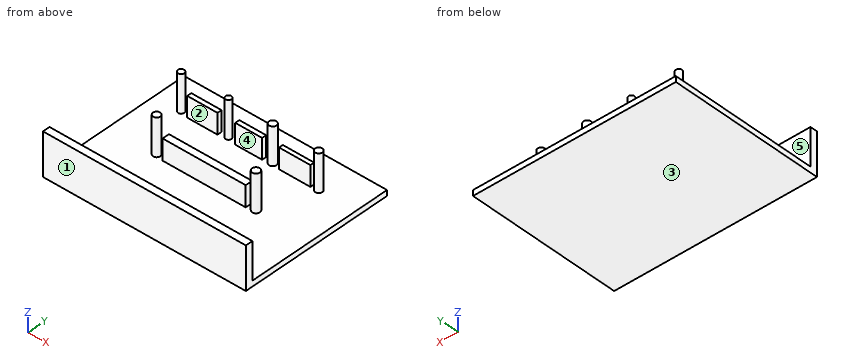
```python
from build123d import *

# Parameters (mm, degrees)
F0_W      = 138.621978
F0_H      = 105.59459
F1_DEPTH  = 3.81
F2_R      = 2.106167
F3_DEPTH  = 25.4
F4_R      = 2.000792
F5_DEPTH  = 25.4
F6_R      = 2.558459
F7_DEPTH  = 25.4
F8_R      = 2.472435
F9_DEPTH  = 25.4
F10_W     = 138.621978
F10_H     = 4.884328
F11_DEPTH = 25.4
F12_R     = 2.472435
F13_DEPTH = 25.4
F14_R     = 2.6519
F15_DEPTH = 25.4
F16_W     = 20.700261
F16_H     = 3.023634
F16_W_2   = 18.374391
F16_W_3   = 21.398022
F16_H_2   = 2.791049
F17_DEPTH = 13.97
F18_W     = 56.751281
F18_H     = 4.768038
F19_DEPTH = 14.224


with BuildPart() as f1:
    # F0 (on Top) → F1 (new body)
    with BuildSketch(Plane.XY):
        with Locations((1.744408, 1.046643)):
            Rectangle(F0_W, F0_H)
    extrude(amount=F1_DEPTH)

    # F2 (on face) → F3 (join)
    with BuildSketch(Plane.XY.offset(3.81)):
        with Locations((-49.192194, 31.515568)):
            Circle(F2_R)
    extrude(amount=F3_DEPTH)

    # F4 (on face) → F5 (join)
    with BuildSketch(Plane.XY.offset(3.81)):
        with Locations((-17.09516, 31.748157)):
            Circle(F4_R)
    extrude(amount=F5_DEPTH)

    # F6 (on face) → F7 (join)
    with BuildSketch(Plane.XY.offset(3.81)):
        with Locations((13.606353, 31.28298)):
            Circle(F6_R)
    extrude(amount=F7_DEPTH)

    # F8 (on face) → F9 (join)
    with BuildSketch(Plane.XY.offset(3.81)):
        with Locations((45.703389, 30.585218)):
            Circle(F8_R)
    extrude(amount=F9_DEPTH)

    # F10 (on face) → F11 (join)
    with BuildSketch(Plane.XY.offset(3.81)):
        with Locations((1.744408, -49.308488)):
            Rectangle(F10_W, F10_H)
    extrude(amount=F11_DEPTH)

    # F12 (on face) → F13 (join)
    with BuildSketch(Plane.XY.offset(3.81)):
        with Locations((-34.5392, -2.90734)):
            Circle(F12_R)
    extrude(amount=F13_DEPTH)

    # F14 (on face) → F15 (join)
    with BuildSketch(Plane.XY.offset(3.81)):
        with Locations((33.376262, -2.90734)):
            Circle(F14_R)
    extrude(amount=F15_DEPTH)

    # F16 (on face) → F17 (join)
    with BuildSketch(Plane.XY.offset(3.81)):
        with Locations((-33.027384, 31.166687)):
            Rectangle(F16_W, F16_H)
        with Locations((-1.395523, 31.166687)):
            Rectangle(F16_W_2, F16_H)
        with Locations((30.120045, 31.050394)):
            Rectangle(F16_W_3, F16_H_2)
    extrude(amount=F17_DEPTH)

    # F18 (on face) → F19 (join)
    with BuildSketch(Plane.XY.offset(3.81)):
        with Locations((-0.34888, -2.384019)):
            Rectangle(F18_W, F18_H)
    extrude(amount=F19_DEPTH)


solid = f1.part
```
Build history of the part. All positions in model axes, mm. Face numbers are marked on the shaded views. A direction names the side the tool comes from. Round coordinates to 2 decimals unless told otherwise and drop trailing zeros. Write each loop counter-clockwise with the first axis right and the second up, starting at its lowest first coordinate (ties: lowest second). Pieces come first, ordered by that corner, then holes. Notation, with made-up numbers: (78, 88) -> (109, 88) arc R15 ccw to (109, 107) -> close; hole circle Ø1 at (-33.75, 32.25). An arc over 180 degrees is marked (long way). Put each result on its own line as item: value.
Item 1: Wall check: probe 1 along Y at (x, z) = (-25.5, 10); probe 2 along Y at (x, z) = (-11, 11.5); probe 3 along X at (y, z) = (-1, 13.75). Give the ranges that are in metal, low to high. Write a range as from..to.
Here are the results:
probe 1: y = -51.75..-46.87, -4.77..0, 29.65..32.68
probe 2: y = -51.75..-46.87, -4.77..0
probe 3: x = -36.11..-32.97, -28.72..28.03, 31.53..35.22
Item 2: Slice it at B-B, the plane x = -40.5. Give the cut face in (y, z).
Here are the results:
outline: (-51.75, 0) -> (53.84, 0) -> (53.84, 3.81) -> (32.68, 3.81) -> (32.68, 17.78) -> (29.65, 17.78) -> (29.65, 3.81) -> (-46.87, 3.81) -> (-46.87, 29.21) -> (-51.75, 29.21) -> close
Item 3: Slice it at A-A, the plane z = 15. Count the separate pieces of the cut face and the enclosed holes in it, plus the area to 3 significant figures.
Here are the results:
separate pieces: 11
enclosed holes: 0
area: 1,230 mm^2
Item 4: Tool access for the marked faces 3, 4 and 5: list every direction of +Z, -Z, +X, -X, +Y, -Y with a clear straight run to the whole face (end or side of a thin tool).
Here are the results:
face 3: -Z, +X, -X, +Y, -Y
face 4: +Z
face 5: +Z, +X, -X
Item 5: Two-plate mould, pull along X, no slides. Class the marked faces 1 and 2: pulls with the +X half, pulls with the -X half, needs draft (parallel to the pull), parting line crosses it, or undercut.
Here are the results:
face 1: needs draft
face 2: undercut
Item 6: Flat gauge pins, fed straight in: P1, Ø2, axis at x = -32, y = 0.5, coming from the +Z side; P2, Ø1.4, axis at x = 27.5, y = 30.5, coming from the +Z side; P3, Ø2.5, axis at x = -8, y = -2, coming from the +Z side. Where does each tip first touch, or does it go through?
Here are the results:
P1: stops at z = 3.81
P2: stops at z = 17.78
P3: stops at z = 18.03
Item 7: Slice it at D-D, the plane y = -14.5. Give the cut face in (x, z).
Here are the results:
outline: (-67.57, 0) -> (71.06, 0) -> (71.06, 3.81) -> (-67.57, 3.81) -> close
Item 8: Slice it at C-C, the plane z = 24.5. Give the cut face in (x, y).
Here are the results:
outline: (-67.57, -51.75) -> (71.06, -51.75) -> (71.06, -46.87) -> (-67.57, -46.87) -> close; circle Ø4.21 at (-49.19, 31.52); circle Ø4.94 at (-34.54, -2.91); circle Ø4 at (-17.1, 31.75); circle Ø5.12 at (13.61, 31.28); circle Ø5.3 at (33.38, -2.91); circle Ø4.94 at (45.7, 30.59)
